```python
from build123d import *

# Parameters (mm, degrees)
BOSS_EXTRUDE1_DEPTH = 1.5875
SKETCH3_R           = 1.1049
SKETCH3_R_2         = 1.651
SKETCH3_R_3         = 1.5875
SKETCH3_R_4         = 0.4826
CUT_EXTRUDE1_DEPTH  = 2.5875
SKETCH4_R           = 0.508
SKETCH4_R_2         = 0.4064
CUT_EXTRUDE2_DEPTH  = 2.5875


with BuildPart() as part:
    # Sketch2 → Boss-Extrude1 (new body)
    with BuildSketch(Plane.XY):
        Polygon((-34.2899492, 26.67), (30.2259492, 26.67), (31.7499492, 25.146), (31.7499492, 13.716), (34.2899492, 11.176), (34.2899492, -21.59), (31.7499492, -24.13), (31.7499492, -26.67), (-34.2899492, -26.67), align=None)
    extrude(amount=-BOSS_EXTRUDE1_DEPTH)

    # Sketch3 → Cut-Extrude1 (cut, through all)
    with BuildSketch(Plane.XY):
        with Locations((-30.4799492, 17.429988)):
            Circle(SKETCH3_R)
        with Locations((-30.4799492, 5.430012)):
            Circle(SKETCH3_R)
        with Locations((-28.6003492, -18.3642)):
            Circle(SKETCH3_R_2)
        with Locations((-25.6031492, -23.368)):
            Circle(SKETCH3_R_2)
        with Locations((-22.6060508, -18.3642)):
            Circle(SKETCH3_R_2)
        with Locations((31.7499492, -19.05)):
            Circle(SKETCH3_R_3)
        with Locations((31.7499492, 8.89)):
            Circle(SKETCH3_R_3)
        with Locations((-19.0500508, 24.13)):
            Circle(SKETCH3_R_3)
        with Locations((-25.769951, 12.679934)):
            Circle(SKETCH3_R_4)
        with Locations((-27.769947, 12.679934)):
            Circle(SKETCH3_R_4)
        with Locations((-27.769947, 10.180066)):
            Circle(SKETCH3_R_4)
        with Locations((-25.769951, 10.180066)):
            Circle(SKETCH3_R_4)
    extrude(amount=-CUT_EXTRUDE1_DEPTH, mode=Mode.SUBTRACT)

    # Sketch4 → Cut-Extrude2 (cut, through all)
    with BuildSketch(Plane.XY):
        with Locations((29.2099492, 24.13)):
            Circle(SKETCH4_R)
        with Locations((26.6699492, 24.13)):
            Circle(SKETCH4_R)
        with Locations((24.1299492, 24.13)):
            Circle(SKETCH4_R)
        with Locations((21.5899492, 24.13)):
            Circle(SKETCH4_R)
        with Locations((19.0499492, 24.13)):
            Circle(SKETCH4_R)
        with Locations((16.5099492, 24.13)):
            Circle(SKETCH4_R)
        with Locations((13.9699492, 24.13)):
            Circle(SKETCH4_R)
        with Locations((11.4299492, 24.13)):
            Circle(SKETCH4_R)
        with Locations((7.3659492, 24.13)):
            Circle(SKETCH4_R)
        with Locations((4.8259492, 24.13)):
            Circle(SKETCH4_R)
        with Locations((2.2859492, 24.13)):
            Circle(SKETCH4_R)
        with Locations((-0.2540508, 24.13)):
            Circle(SKETCH4_R)
        with Locations((-2.7940508, 24.13)):
            Circle(SKETCH4_R)
        with Locations((-5.3340508, 24.13)):
            Circle(SKETCH4_R)
        with Locations((-7.8740508, 24.13)):
            Circle(SKETCH4_R)
        with Locations((-10.4140508, 24.13)):
            Circle(SKETCH4_R)
        with Locations((28.5749492, -6.477)):
            Circle(SKETCH4_R_2)
        with Locations((26.0349492, -6.477)):
            Circle(SKETCH4_R_2)
        with Locations((23.4949492, -6.477)):
            Circle(SKETCH4_R_2)
        with Locations((20.9549492, -6.477)):
            Circle(SKETCH4_R_2)
        with Locations((18.4149492, -6.477)):
            Circle(SKETCH4_R_2)
        with Locations((15.8749492, -6.477)):
            Circle(SKETCH4_R_2)
        with Locations((13.3349492, -6.477)):
            Circle(SKETCH4_R_2)
        with Locations((10.7949492, -6.477)):
            Circle(SKETCH4_R_2)
        with Locations((8.2549492, -6.477)):
            Circle(SKETCH4_R_2)
        with Locations((5.7149492, -6.477)):
            Circle(SKETCH4_R_2)
        with Locations((3.1749492, -6.477)):
            Circle(SKETCH4_R_2)
        with Locations((0.6349492, -6.477)):
            Circle(SKETCH4_R_2)
        with Locations((-1.9050508, -6.477)):
            Circle(SKETCH4_R_2)
        with Locations((-4.4450508, -6.477)):
            Circle(SKETCH4_R_2)
        with Locations((28.5749492, -14.097)):
            Circle(SKETCH4_R_2)
        with Locations((26.0349492, -14.097)):
            Circle(SKETCH4_R_2)
        with Locations((23.4949492, -14.097)):
            Circle(SKETCH4_R_2)
        with Locations((20.9549492, -14.097)):
            Circle(SKETCH4_R_2)
        with Locations((18.4149492, -14.097)):
            Circle(SKETCH4_R_2)
        with Locations((15.8749492, -14.097)):
            Circle(SKETCH4_R_2)
        with Locations((13.3349492, -14.097)):
            Circle(SKETCH4_R_2)
        with Locations((10.7949492, -14.097)):
            Circle(SKETCH4_R_2)
        with Locations((8.2549492, -14.097)):
            Circle(SKETCH4_R_2)
        with Locations((5.7149492, -14.097)):
            Circle(SKETCH4_R_2)
        with Locations((3.1749492, -14.097)):
            Circle(SKETCH4_R_2)
        with Locations((0.6349492, -14.097)):
            Circle(SKETCH4_R_2)
        with Locations((-1.9050508, -14.097)):
            Circle(SKETCH4_R_2)
        with Locations((-4.4450508, -14.097)):
            Circle(SKETCH4_R_2)
        with Locations((29.2099492, -24.13)):
            Circle(SKETCH4_R)
        with Locations((11.4299492, -24.13)):
            Circle(SKETCH4_R)
        with Locations((26.6699492, -24.13)):
            Circle(SKETCH4_R)
        with Locations((8.8899492, -24.13)):
            Circle(SKETCH4_R)
        with Locations((24.1299492, -24.13)):
            Circle(SKETCH4_R)
        with Locations((6.3499492, -24.13)):
            Circle(SKETCH4_R)
        with Locations((21.5899492, -24.13)):
            Circle(SKETCH4_R)
        with Locations((3.8099492, -24.13)):
            Circle(SKETCH4_R)
        with Locations((19.0499492, -24.13)):
            Circle(SKETCH4_R)
        with Locations((1.2699492, -24.13)):
            Circle(SKETCH4_R)
        with Locations((16.5099492, -24.13)):
            Circle(SKETCH4_R)
        with Locations((-1.2700508, -24.13)):
            Circle(SKETCH4_R)
        with Locations((-13.4620508, 20.828)):
            Circle(SKETCH4_R)
        with Locations((-13.4620508, 18.288)):
            Circle(SKETCH4_R)
        with Locations((-16.0020508, 18.288)):
            Circle(SKETCH4_R)
        with Locations((-16.0020508, 20.828)):
            Circle(SKETCH4_R)
        with Locations((-18.5420508, 18.288)):
            Circle(SKETCH4_R)
        with Locations((-18.5420508, 20.828)):
            Circle(SKETCH4_R)
        with Locations((31.8901572, -1.320038)):
            Circle(SKETCH4_R)
        with Locations((29.3501572, -1.320038)):
            Circle(SKETCH4_R)
        with Locations((29.3501572, 1.219962)):
            Circle(SKETCH4_R)
        with Locations((31.8901572, 1.219962)):
            Circle(SKETCH4_R)
        with Locations((29.3501572, 3.759962)):
            Circle(SKETCH4_R)
        with Locations((31.8901572, 3.759962)):
            Circle(SKETCH4_R)
    extrude(amount=-CUT_EXTRUDE2_DEPTH, mode=Mode.SUBTRACT)


solid = part.part
```
Could you check a few things on this model? Use its own coordinates, in mm. A direction names the side the tool comes from. Round coordinates to 2 decimals unless told otherwise and drop trailing zeros. Order: outer loops, then holes, each group sorted by start corner. A loop starts at its lowest first (then second) coordinate and runs counter-clockwise, first axis right, second up. Notation, with made-up numbers: M 13,54.25 L 26,54.25 A8 cw 26,62.25 Z; hole C -35,4.25 d6. An arc over 180 degrees is marked long. One line per question, with ' | ' between items. Start each with the question number.
(1) Suppose I cut it at A-A on y = 8.89. List the corners of the cut face in (x, z) for me, then the cut area to 3 significant figures.
(2) Suppose I cut it at C-C on z = -1.1. Count the separate pieces of the cut face and the enclosed holes in it, then the cut area to 3 significant figures.
(3) For faces 1 (the face through (31.75, 20, -1)), 2 (the face through (31.75, -25, -1)), 3 (the face through (-23.916, -19.369, -0.783)), which set-ups out of +Z, -Z, +X, -X, +Y, -Y let a thin tool reach every point of the face, with its end or its side?
(4) Thinking about a two-plate mould opening in Y: for faces 4 (the face through (-1, -26.67, -1)), 5 (the face through (0, 0, 0)), 6 (the face through (-31.584, 17.479, -0.783)), which applies, +Y half, -Y half, draft (parallel to the pull), parting line (faces both ways), or undercut?
(5) For P1, Ø0.6, axis at x = -18.54, y = 20.83, coming from the -Z side, with a flat end and sliding along its axis, tell me the tip position at first contact or that it passes through.
(6) Suppose I cut it at B-B on y = -22.5. List the corners of the cut face in (x, z) for me, then the cut area to 3 significant figures.
(7) Please list where these lines run through material, in increasing order: line 1 along Y through (x, z) = (-4.5, -0.45); line 2 along Y through (x, z) = (-25.5, -0.45); line 3 along X through (y, z) = (5.5, -1.05).
Geometry results:
1) outline: M -34.29,-1.59 L 30.16,-1.59 L 30.16,0 L -34.29,0 Z; M 33.34,-1.59 L 34.29,-1.59 L 34.29,0 L 33.34,0 Z | area: 104 mm²
2) separate pieces: 1 | enclosed holes: 80 | area: 3,500 mm²
3) face 1: +Z, -Z, +X, +Y | face 2: +Z, -Z, +X, -Y | face 3: +Z, -Z
4) face 4: -Y half | face 5: draft | face 6: undercut
5) P1: through
6) outline: M -34.29,-1.59 L -27.01,-1.59 L -27.01,0 L -34.29,0 Z; M -24.2,-1.59 L 33.38,-1.59 L 33.38,0 L -24.2,0 Z | area: 103 mm²
7) line 1: -26.67 to -14.5, -13.69 to -6.88, -6.07 to 26.67 | line 2: -26.67 to -25.02, -21.72 to 9.78, 10.58 to 12.28, 13.08 to 26.67 | line 3: -34.29 to -31.58, -29.38 to 34.29
